The model under review builds one solid part; all positions refer to its coordinate system, in mm. A direction names the side the tool comes from. Round coordinates to 2 decimals unless told otherwise and drop trailing zeros. Loops run counter-clockwise (first coordinate to the right, second up) from the corner with the lowest first, then second, coordinate; pieces in that order, holes last. Notation, with made-up numbers: (41, 80) - (94, 80) arc R26 cw to (94, 111) - close; hole circle Ø11 at (-29, -36). An arc over 180 degrees is marked (long way). Answer as CSV lines item,"result".
from build123d import *

# Parameters (mm, degrees)
SKETCH1_W                 = 35.8902
SKETCH1_H                 = 35.8902
BASE_EXTRUDE_DEPTH        = 101.6
HOLE1_START               = -20.6375
HOLE1_OUTLINE_R           = 7.14375
HOLE1_DEPTH               = 41.275
CIRPATTERN2_COUNT         = 2
CIRPATTERN2_ANGLE         = 90
LPATTERN1_COUNT           = 2
LPATTERN1_PITCH           = 47.625
LPATTERN1_START           = -20.6375
LPATTERN1_COPY_1_SKETCH_R = 7.14375
LPATTERN1_COPY_1_DEPTH    = 41.275


# Read off the part's stored shape, not the designer's step: Hole1
with BuildPart() as part:
    # Sketch1 → Base-Extrude (new body)
    with BuildSketch(Plane.XY):
        with BuildLine():
            Line((-20.6375, 17.9451), (-20.6375, -17.9451))
            ThreePointArc((-20.6375, -17.9451), (-19.848914298, -19.848914298), (-17.9451, -20.6375))
            Line((-17.9451, -20.6375), (17.9451, -20.6375))
            ThreePointArc((17.9451, -20.6375), (19.848914298, -19.848914298), (20.6375, -17.9451))
            Line((20.6375, -17.9451), (20.6375, 17.9451))
            ThreePointArc((20.6375, 17.9451), (19.848914298, 19.848914298), (17.9451, 20.6375))
            Line((17.9451, 20.6375), (-17.9451, 20.6375))
            ThreePointArc((-17.9451, 20.6375), (-19.848914298, 19.848914298), (-20.6375, 17.9451))
        make_face()
        Rectangle(SKETCH1_W, SKETCH1_H, mode=Mode.SUBTRACT)
    extrude(amount=BASE_EXTRUDE_DEPTH)

    # Hole1 outline → Hole1 (cut)
    with BuildSketch(Plane(origin=(0, 0, 0), x_dir=(1, 0, 0), z_dir=(0, 1, 0)).offset(HOLE1_START)):
        with Locations((0, -23.8125)):
            Circle(HOLE1_OUTLINE_R)
    hole1 = extrude(amount=HOLE1_DEPTH, mode=Mode.SUBTRACT)

    # CirPattern2: Hole1 ×2 about axis
    cirpattern2_axis = Axis((0, 0, -50), (0, 0, 1))
    for i in range(1, CIRPATTERN2_COUNT):
        add(hole1.rotate(cirpattern2_axis, i * CIRPATTERN2_ANGLE / (CIRPATTERN2_COUNT - 1)), mode=Mode.SUBTRACT)

    # LPattern1: Hole1 ×2
    with Locations(*[(0, 0, i * LPATTERN1_PITCH) for i in range(1, LPATTERN1_COUNT)]):
        add(hole1, mode=Mode.SUBTRACT)

    # LPattern1 copy 1 sketch → LPattern1 copy 1 (cut)
    with BuildSketch(Plane(origin=(0, 0, 47.625), x_dir=(0, 1, 0), z_dir=(-1, 0, 0)).offset(LPATTERN1_START)):
        with Locations((0, -23.8125)):
            Circle(LPATTERN1_COPY_1_SKETCH_R)
    extrude(amount=LPATTERN1_COPY_1_DEPTH, mode=Mode.SUBTRACT)


solid = part.part
1. Take a section at A-A (y = -13). State the section outline as (x, z) points, plus the area to 3 significant figures.
Numbers:
outline,"(-20.64, 0) - (-17.95, 0) - (-17.95, 101.6) - (-20.64, 101.6) - close; (17.95, 0) - (20.64, 0) - (20.64, 101.6) - (17.95, 101.6) - close"
area,"547 mm²"
2. Take a section at B-B (z = 95.5). State the section outline as (x, y) points, plus the area to 3 significant figures.
Numbers:
outline,"(-20.64, -17.95) arc R2.69 ccw to (-17.95, -20.64) - (17.95, -20.64) arc R2.69 ccw to (20.64, -17.95) - (20.64, 17.95) arc R2.69 ccw to (17.95, 20.64) - (-17.95, 20.64) arc R2.69 ccw to (-20.64, 17.95) - close; hole (-17.95, -17.95) - (17.95, -17.95) - (17.95, 17.95) - (-17.95, 17.95) - close"
area,"409 mm²"
3. Clearance check with a flat-ended pin moving along its axis: pin 1 (13 mm diameter, centred on x = 0, z = 71.44, fed in from +Y). State where the tip first meets the part, or that it passes through.
Numbers:
pin 1,"passes through"
4. Tool access review of faces 1 (the face through (0, -17.945, 50)), 2 (the face through (-1.549, 19.272, 30.786)): name each direction out of +Z, -Z, +X, -X, +Y, -Y from which nothing blocks a thin tool from reaching the whole face with its end or side.
Numbers:
face 1,"+Z, -Z"
face 2,"+Y, -Y"
5. Take a section at D-D (x = -1.5). State the section outline as (y, z) points, plus the area to 3 significant figures.
Numbers:
outline,"(-20.64, 0) - (-17.95, 0) - (-17.95, 16.83) - (-20.64, 16.83) - close; (-20.64, 30.8) - (-17.95, 30.8) - (-17.95, 64.45) - (-20.64, 64.45) - close; (-20.64, 78.42) - (-17.95, 78.42) - (-17.95, 101.6) - (-20.64, 101.6) - close; (17.95, 0) - (20.64, 0) - (20.64, 16.83) - (17.95, 16.83) - close; (17.95, 30.8) - (20.64, 30.8) - (20.64, 64.45) - (17.95, 64.45) - close; (17.95, 78.42) - (20.64, 78.42) - (20.64, 101.6) - (17.95, 101.6) - close"
area,"397 mm²"
6. Wall thickness on probe 1 along Z at (x, y) = (-19.05, 0); probe 2 along Y at (x, z) = (5.5, 78.5): over which ranges is each line inside the solid? List them lowest first.
Numbers:
probe 1,"z = 0 to 16.67, 30.96 to 64.29, 78.58 to 101.6"
probe 2,"y = -20.64 to -17.95, 17.95 to 20.64"
7. Draft analysis for pull direction Z (two halves, no side actions). For faces 3 (the face through (-1.549, -19.31, 30.786)), 4 (the face through (20.638, 0, 50)), 5 (the face through (-19, 0, 101.6)), 6 (the face through (-19, 0, 0)), state which applies: +Z half, -Z half, draft (parallel to the pull), parting line (faces both ways), or undercut.
Numbers:
face 3,"undercut"
face 4,"draft"
face 5,"+Z half"
face 6,"-Z half"
